Could you check a few things on this model? Use its own coordinates, in mm. Give positions to 0.01 mm unless a question says otherwise; leave off trailing zeros. Loops run counter-clockwise (first coordinate to the right, second up) from the corner with the lowest first, then second, coordinate; pieces in that order, holes last. Notation, with made-up numbers: (71.25, 2.5) - (94.25, 2.5) arc R10 cw to (94.25, 6.5) - close; hole circle Ø3 at (69.25, 16.25). An arc over 180 degrees is marked (long way). One line per item, written item: value. Start each with the question number.
Q1. I want a section at A-A (y = 0). Please give me the cut outline in (x, z).
Q2. If we mould it in two halves opening along Y, with no side actions, what happens to faces 1 (the face through (-34.685, 156.195, 4.93)), 2 (the face through (33, 109, 0)), 3 (the face through (-44.026, 118.302, 4.93))? For each: released by +Y, released by -Y, zero draft, split by the parting line, or undercut.
Q3. If I drill on line 1 (Y direction, x = -122, z = 4.25); line 2 (Y direction, x = -124.5, z = 3.5); line 3 (X direction, y = 94, z = 4.5), over which ranges is the centre line in solid material (lowest first)? Write a range as from..to.
Q4. I want a section at D-D (y = -135.5). Please give me the cut outline in (x, z).
Q5. I want a section at C-C (z = 5.5). Count the separate pieces of the cut face and the enclosed holes in it, then the cut area to 3 significant figures.
Q6. I'm going to push flat-ended pins straight in: P1, Ø6, axis at x = 9.5, z = 7.5, coming from the -Y side; P2, Ø2, axis at x = -3, z = 2.5, coming from the -Y side; P3, Ø1.5, axis at y = 81.5, z = 2.5, coming from the +X side. Where does each tip first touch, or does it pass through?
Autodesk Inventor part; units mm, degrees
ref_plane "YZ Plane" through (0, 0, 0) normal (1, 0, 0) x (0, 1, 0)
ref_plane "XZ Plane" through (0, 0, 0) normal (0, 1, 0) x (-1, 0, 0)
ref_plane "XY Plane" through (0, 0, 0) normal (0, 0, 1) x (1, 0, 0)
sketch "Эскиз1" plane through (0, 0, 0) normal (0, 0, 1) x (1, 0, 0)
  circle A0 centre (0, 0) radius 112.5
  circle A1 centre (0, 0) radius 160
  dimension "d0" = 225
  dimension "d1" = 320
extrude "Выдавливание1" add sketch "Эскиз1" along normal blind 10
sketch "Эскиз2" plane through (0, 0, 10) normal (0, 0, 1) x (1, 0, 0)
  line L0 (0, 0) -> (120.1043, 49.7488)
  line L1 (-224, 0) -> (224, 0)
  dimension "d4" = 130
  dimension "d5" = 22.5
hole "Отверстие1" at (120.1043, 49.7488, 10) direction (0, 0, -1) diameter 12 end through all
pattern_circular "Круговой массив1" count 8 over 360 about axis through (0, 0, 0) along (0, 0, 1) of "Отверстие1"
properties part number "Придав перегородки1" material "Сталь, высокопрочная, низколегированная"
Worked answers:
1. outline: (-160, 0) - (-112.5, 0) - (-112.5, 10) - (-160, 10) - close; (112.5, 0) - (160, 0) - (160, 10) - (112.5, 10) - close
2. face 1: split by the parting line
2. face 2: zero draft
2. face 3: undercut
3. line 1: y = -103.52..-55.44, -44.06..44.06, 55.44..103.52
3. line 2: y = -100.5..-53.83, -45.66..45.67, 53.83..100.5
3. line 3: x = -129.48..-61.81, 61.81..129.48
4. outline: (-85.09, 0) - (85.09, 0) - (85.09, 10) - (-85.09, 10) - close
5. separate pieces: 1
5. enclosed holes: 9
5. area: 39,800 mm²
6. P1: stops at y = -159.87
6. P2: stops at y = -159.99
6. P3: stops at x = 138.13
